For this review, take the finished solid that the model builds, in its own axes (mm). Face numbers are marked on the shaded views. Round coordinates to 2 decimals unless told otherwise and drop trailing zeros. Write each loop counter-clockwise with the first axis right and the second up, starting at its lowest first coordinate (ties: lowest second). Pieces come first, ordered by that corner, then holes. Notation, with made-up numbers: M 28,-22 L 38,-22 A20 ccw 38,-10 Z; hole C -19.5,68 d7. An arc over 180 degrees is marked long. Write each question's results on one line, items separated by ' | '. Start each with the question number.
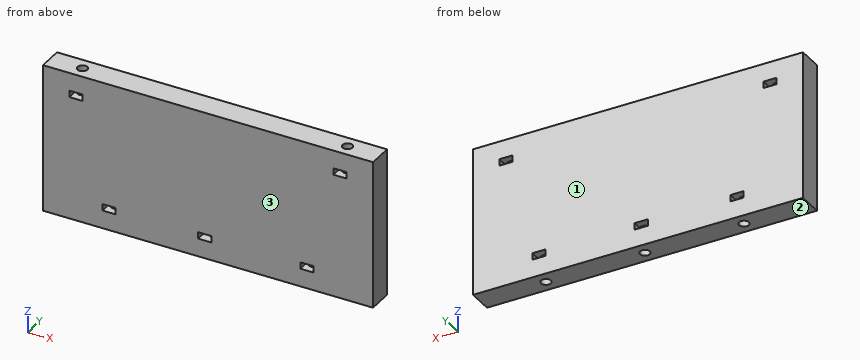
```python
from build123d import *

# Parameters (mm, degrees)
SKETCH1_W           = 200
SKETCH1_H           = 90
SKETCH1_W_2         = 8
SKETCH1_H_2         = 4
BOSS_EXTRUDE1_DEPTH = 15
SKETCH2_R           = 3
CUT_EXTRUDE1_DEPTH  = 20
SKETCH3_R           = 3
CUT_EXTRUDE2_DEPTH  = 20


with BuildPart() as part:
    # Sketch1 → Boss-Extrude1 (new body)
    with BuildSketch(Plane(origin=(0, 0, 0), x_dir=(1, 0, 0), z_dir=(0, 1, 0))):
        with Locations((-5.131403118, 11.792873051)):
            Rectangle(SKETCH1_W, SKETCH1_H)
        with Locations((54.868596882, 43.860843617)):
            Rectangle(SKETCH1_W_2, SKETCH1_H_2, mode=Mode.SUBTRACT)
        with Locations((-65.131403118, 43.860843617)):
            Rectangle(SKETCH1_W_2, SKETCH1_H_2, mode=Mode.SUBTRACT)
        with Locations((-7.131403118, 43.860843617)):
            Rectangle(SKETCH1_W_2, SKETCH1_H_2, mode=Mode.SUBTRACT)
        with Locations((74.868596882, -20.275097514)):
            Rectangle(SKETCH1_W_2, SKETCH1_H_2, mode=Mode.SUBTRACT)
        with Locations((-85.131403118, -20.275097514)):
            Rectangle(SKETCH1_W_2, SKETCH1_H_2, mode=Mode.SUBTRACT)
    extrude(amount=BOSS_EXTRUDE1_DEPTH)

    # Sketch2 → Cut-Extrude1 (cut)
    with BuildSketch(Plane(origin=(0, 0, -56.792873051), x_dir=(-1, 0, 0), z_dir=(0, 0, -1))):
        with Locations((-54.868596882, 7.5)):
            Circle(SKETCH2_R)
        with Locations((5.131403118, 7.5)):
            Circle(SKETCH2_R)
        with Locations(Location((65.131403118, 7.5, 0), (0, 0, 180))):
            Circle(SKETCH2_R)
    extrude(amount=-CUT_EXTRUDE1_DEPTH, mode=Mode.SUBTRACT)

    # Sketch3 → Cut-Extrude2 (cut)
    with BuildSketch(Plane.XY.offset(33.207126949)):
        with Locations((-85.445029849, 7.5)):
            Circle(SKETCH3_R)
        with Locations((75.182223613, 7.5)):
            Circle(SKETCH3_R)
    extrude(amount=-CUT_EXTRUDE2_DEPTH, mode=Mode.SUBTRACT)


solid = part.part
```
Item 1: We need section A-A on x = -6. State the section outline as (y, z) points.
Item 2: For probe 1 along X at (y, z) = (3.5, -43.5); probe 2 along X at (y, z) = (9.5, 19); probe 3 along Z at (x, y) = (-63.5, 1.75), list the stretches that pass through material, from the lowest coordinate up.
Item 3: Insertion check: P1, Ø5, axis at x = 75.18, y = 7.5, coming from the +Z side. The pin has a flat end and moves straight along its axis. Give the tip position at first contact, or say it passes through.
Item 4: Mouldability with a two-part tool opening along Y and no side actions: class the marked faces 1, 2 and 3 as pulls with the +Y half, pulls with the -Y half, needs draft (parallel to the pull), parting line crosses it, or undercut.
Numbers:
1) outline: M 0,-56.79 L 4.63,-56.79 L 4.63,-45.86 L 0,-45.86 Z; M 0,-41.86 L 4.63,-41.86 L 4.63,-36.79 L 10.37,-36.79 L 10.37,-41.86 L 15,-41.86 L 15,33.21 L 0,33.21 Z; M 10.37,-56.79 L 15,-56.79 L 15,-45.86 L 10.37,-45.86 Z
2) probe 1: x = -105.13 to -69.13, -61.13 to -11.13, -3.13 to 50.87, 58.87 to 94.87 | probe 2: x = -105.13 to -89.13, -81.13 to 70.87, 78.87 to 94.87 | probe 3: z = -56.79 to -45.86, -41.86 to 33.21
3) P1: stops at z = 13.21
4) face 1: pulls with the +Y half | face 2: needs draft | face 3: pulls with the -Y half
